Job drawing, mm, ordinate dimensions from the low corner. One solid piece. A direction names the side the tool comes from. Give positions to 0.01 mm unless a question says otherwise; leave off trailing zeros. Write each loop counter-clockwise with the first axis right and the second up, starting at its lowest first coordinate (ties: lowest second). Pieces come first, ordered by that corner, then holes. Notation, with made-up numbers: (-5.75, 61.25) - (7.25, 61.25) arc R29 ccw to (7.25, 87.25) - close; hole circle Ø2 at (61, 26). An arc over 180 degrees is marked (long way). Put each result on its own line as item: value. Start each with the question number.
1. Drop flat-ended pins along their axis: pin 1 (1 mm diameter, centred on y = 4, z = 2, fed in from +X); pin 2 (1.5 mm diameter, centred on y = 3.5, z = 1, fed in from -X); pin 3 (1.2 mm diameter, centred on y = 2.5, z = 1.5, fed in from -X) (1 decimal). Give the stop position or say it passes through.
2. Cut at A-A on z = 2.05. List the corners of the cut face in (x, y) (1 decimal).
3. Tool access for the marked faces 1, 2 and 3: list every direction of +Z, -Z, +X, -X, +Y, -Y with a clear straight run to the whole face (end or side of a thin tool).
4. Wall check: line 1 (Y direction, x = 1.65, z = 2.3) (1 decimal); line 2 (X direction, y = 3, z = 2.65) (1 decimal); line 3 (Y direction, x = 2.2, z = 1.9) (1 decimal). Give the ranges that are in metal, low to high.
5. Mould opens along Y. For the marked faces 4, 5, 6 and 7 say: +Y half, -Y half, draft (parallel to the pull), parting line (faces both ways), or undercut.
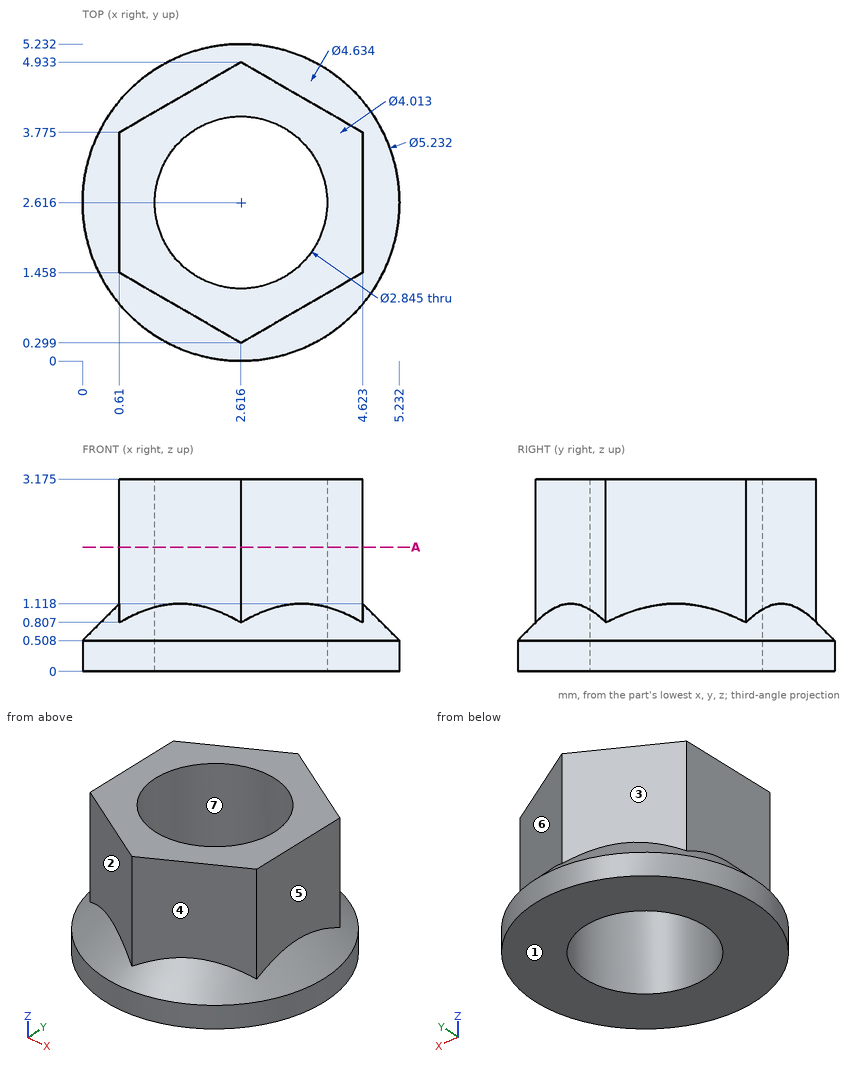
Report:
1. pin 1: stops at x = 4.62
1. pin 2: stops at x = 0.02
1. pin 3: stops at x = 0.4
2. outline: (0.6, 1.5) - (2.6, 0.3) - (4.6, 1.5) - (4.6, 3.8) - (2.6, 4.9) - (0.6, 3.8) - close; hole circle Ø2.8 at (2.6, 2.6)
3. face 1: -Z, +X, -X, +Y, -Y
3. face 2: +Z, -X, -Y
3. face 3: +Z, -X, +Y
4. line 1: y = 0.9 to 1.6, 3.7 to 4.4
4. line 2: x = 0.6 to 1.2, 4 to 4.6
4. line 3: y = 0.5 to 1.3, 4 to 4.7
5. face 4: -Y half
5. face 5: draft
5. face 6: +Y half
5. face 7: undercut
